Autodesk Inventor part; units mm, degrees
ref_plane "Work Plane1" through (0, 0, -6) normal (0, 0, -1) x (-1, 0, 0)
ref_plane "YZ Plane" through (0, 0, 0) normal (1, 0, 0) x (0, 1, 0)
ref_plane "XZ Plane" through (0, 0, 0) normal (0, 1, 0) x (-1, 0, 0)
sketch "スケッチ2" plane through (0, 0, 0) normal (0, 0, 1) x (1, 0, 0)
  line L0 (-13.5609, 243.4507) -> (-13.5609, 273.4507)
  line L1 (-13.5609, 273.4507) -> (136.4391, 273.4507)
  arc A0 (136.4391, 243.4507) -> (136.4391, 273.4507) centre (136.4391, 258.4507) ccw
  line L2 (136.4391, 243.4507) -> (-13.5609, 243.4507)
  point P0 (0, 0)
  dimension "d15" = 15
  dimension "d48" = 150
extrude "押し出し2" add sketch "スケッチ2" against normal blind 12
sketch "スケッチ3" plane through (0, 0, 0) normal (0, 0, 1) x (1, 0, 0)
  arc A0 (136.4391, 273.4507) -> (136.4391, 243.4507) centre (136.4391, 258.4507) ccw
  point P0 (86.4391, 253.4507)
  point P1 (66.4391, 253.4507)
  dimension "d4" = 20
  dimension "d5" = 50
  dimension "d6" = 5
hole "穴1" at (86.4391, 253.4507, 0) at (66.4391, 253.4507, 0) direction (0, 0, -1) diameter 8 end through all
sketch "スケッチ4" plane through (0, 0, -12) normal (0, 0, -1) x (-1, 0, 0)
  arc A0 (-136.4391, 273.4507) -> (-136.4391, 243.4507) centre (-136.4391, 258.4507) ccw
hole "穴2" at (136.4391, 258.4507, -12) direction (0, 0, 1) diameter 14 end through all
sketch "スケッチ7" plane through (0, 0, 0) normal (0, 0, 1) x (1, 0, 0)
  arc A0 (136.4391, 243.4507) -> (136.4391, 273.4507) centre (136.4391, 258.4507) ccw
  line L0 (136.4391, 273.4507) -> (-13.5609, 273.4507)
  line L1 (-13.5609, 243.4507) -> (136.4391, 243.4507)
  line L2 (-13.5609, 273.4507) -> (-13.5609, 283.4507)
  line L3 (-13.5609, 283.4507) -> (106.4391, 283.4507)
  line L4 (106.4391, 283.4507) -> (140.879, 272.7786)
  dimension "d49" = 10
  dimension "d50" = 120
extrude "押し出し3" add sketch "スケッチ7" against normal up to surface (12 mm away)
sketch "スケッチ8" plane through (0, 0, 0) normal (0, 0, 1) x (1, 0, 0)
  line L0 (-13.5609, 243.4507) -> (41.4391, 243.4507)
  line L1 (41.4391, 243.4507) -> (41.4391, 253.4507)
  line L2 (41.4391, 253.4507) -> (-13.5609, 253.4507)
  line L3 (-13.5609, 253.4507) -> (-13.5609, 243.4507)
  dimension "d53" = 10
  dimension "d54" = 55
extrude "押し出し4" cut sketch "スケッチ8" against normal through all
sketch "スケッチ9" plane through (-13.5609, 253.4507, 0) normal (0, -1, 0) x (1, 0, 0)
  line L0 (55, 0) -> (55, -12)
  line L1 (0, -12) -> (0, 0)
  line L2 (0, -6) -> (55, -6)
  point P0 (10, -6)
  point P1 (45, -6)
  dimension "d57" = 10
  dimension "d58" = 35
hole "穴5" at (-3.5609, 253.4507, -6) at (31.4391, 253.4507, -6) direction (0, 1, 0) diameter 6.6 end through all
chamfer "面取り1" distance 5 angle 45 1 edges at (-13.5609, 283.4507, -6)
ref_plane "Work Plane1" through (0, 0, -6) normal (0, 0, -1) x (-1, 0, 0)
properties part number "210-109c" material "STEEL - HIGH GRADE ALLOY"
Check sheet for the modelled part. Datum: model origin and axes. Units: mm. A direction names the side the tool comes from. Give positions to 0.01 mm unless a question says otherwise; leave off trailing zeros. Order: outer loops, then holes, each group sorted by start corner. A loop starts at its lowest first (then second) coordinate and runs counter-clockwise, first axis right, second up. Notation, with made-up numbers: M -36.75,2.5 L -11.75,2.5 A20 cw -11.75,26.5 Z; hole C 47.25,85.25 d5. An arc over 180 degrees is marked long. Answer as CSV lines item,"result". Start each with the question number.
Item 1: Mould release check, pull along Z, two halves, no side actions. Record for faces 3 (the face through (68, 264, -12)), 4 (the face through (28.167, 268.661, -5.57)), 5 (the face through (66.263, 257.447, -6.084)): +Z half, -Z half, draft (parallel to the pull), parting line (faces both ways), or undercut.
Item 2: Cross-section at D-D on y = 271. Enter the section's corners in (x, z), plus the area to 3 significant figures.
Item 3: Tool access check on faces 1 (the face through (41.439, 248, -6)), 2 (the face through (90, 243.451, -6)). Record the directions out of +Z, -Z, +X, -X, +Y, -Y that give a thin tool (end or side, any length) a straight path to the whole face; none if there is none.
Item 4: Cross-section at A-A on z = -5.5. Enter the section's corners in (x, y), plus the area to 3 significant figures.
Item 5: Cross-section at B-B on y = 263. Enter the section's corners in (x, z).
Item 6: Cross-section at C-C on x = 2.5. Enter the section's corners in (y, z), plus the area to 3 significant figures.
Item 7: Thickness scan on line 1 (X direction, y = 253.5, z = -1.75); line 2 (X direction, y = 267.25, z = -6); line 3 (X direction, y = 262.25, z = -6). Record the ranges inside material, lowest first. Write a range as [from, to].
Established:
1,face 3,"-Z half"
1,face 4,"undercut"
1,face 5,"draft"
2,outline,"M -13.56,-12 L 144.66,-12 L 144.66,0 L -13.56,0 Z; hole C -3.56,-6 d6.6; hole C 31.44,-6 d6.6"
2,area,"1,830 mm^2"
3,face 1,"+Z, -Z, -X, -Y"
3,face 2,"+Z, -Z, +X, -X, -Y"
4,outline,"M -13.56,253.45 L -6.82,253.45 L -6.82,283.45 L -8.56,283.45 L -13.56,278.45 Z; M -0.3,253.45 L 28.18,253.45 L 28.18,283.45 L -0.3,283.45 Z; M 34.7,253.45 L 41.44,253.45 L 41.44,243.45 L 136.44,243.45 A15 ccw 140.88,272.78 L 106.44,283.45 L 34.7,283.45 Z; hole C 66.44,253.45 d8; hole C 86.44,253.45 d8; hole C 136.44,258.45 d14"
4,area,"5,010 mm^2"
5,outline,"M -13.56,-12 L 131.12,-12 L 131.12,0 L -13.56,0 Z; M 141.76,-12 L 150.73,-12 L 150.73,0 L 141.76,0 Z; hole C -3.56,-6 d6.6; hole C 31.44,-6 d6.6"
6,outline,"M 253.45,-12 L 283.45,-12 L 283.45,0 L 253.45,0 Z"
6,area,"360 mm^2"
7,line 1,"x = [-13.56, 62.44], [70.44, 82.44], [90.44, 131.49], [141.39, 150.6]"
7,line 2,"x = [-13.56, -6.86], [-0.26, 28.14], [34.74, 148.59]"
7,line 3,"x = [-13.56, -6.86], [-0.26, 28.14], [34.74, 130.56], [142.32, 150.95]"
